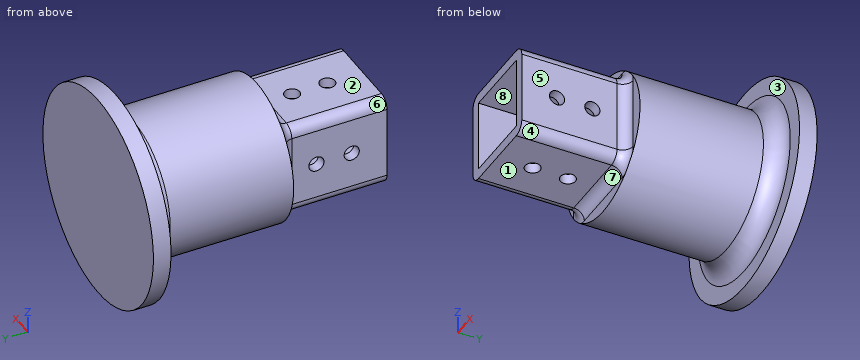
```python
from build123d import *

# Parameters (mm, degrees)
SKETCH_1_R          = 20
SKETCH_1_W          = 20.5
SKETCH_1_H          = 20.5
EXTRUDE_1_DEPTH     = 30
SKETCH_5_R          = 20
EXTRUDE_3_DEPTH     = 10
SKETCH_3_W          = 26.5
SKETCH_3_H          = 26.5
SKETCH_3_W_2        = 20.5
SKETCH_3_H_2        = 20.5
EXTRUDE_4_DEPTH     = 30
SKETCH_6_R          = 2.15
CUT_EXTRUDE_1_DEPTH = 30
SKETCH_7_R          = 2.15
CUT_EXTRUDE_2_DEPTH = 30
FILLET_1_R          = 3
FILLET_2_R          = 3
FILLET_3_R          = 3
FILLET_4_R          = 3
FILLET_5_R          = 3
SKETCH_11_R         = 30
EXTRUDE_5_DEPTH     = 5
FILLET_6_R          = 5


with BuildPart() as part:
    # 草图1 → 凸台-拉伸1 (new body)
    with BuildSketch(Plane(origin=(0, 0, 0), x_dir=(1, 0, 0), z_dir=(0, 1, 0))):
        with Locations(Location((0, 0, 0), (0, 0, 270))):
            Circle(SKETCH_1_R)
        Rectangle(SKETCH_1_W, SKETCH_1_H, mode=Mode.SUBTRACT)
    extrude(amount=EXTRUDE_1_DEPTH)

    # 草图5 → 凸台-拉伸3 (add)
    with BuildSketch(Plane(origin=(0, 30, 0), x_dir=(1, 0, 0), z_dir=(0, 1, 0))):
        with Locations(Location((0, 0, 0), (0, 0, 270))):
            Circle(SKETCH_5_R)
    extrude(amount=EXTRUDE_3_DEPTH)

    # 草图3 → 凸台-拉伸4 (add)
    with BuildSketch(Plane.XZ):
        Rectangle(SKETCH_3_W, SKETCH_3_H)
        Rectangle(SKETCH_3_W_2, SKETCH_3_H_2, mode=Mode.SUBTRACT)
    extrude(amount=EXTRUDE_4_DEPTH)

    # 草图6 → 切除-拉伸1 (cut)
    with BuildSketch(Plane.XY.offset(13.25)):
        with Locations((0, -10)):
            Circle(SKETCH_6_R)
        with Locations((0, -20)):
            Circle(SKETCH_6_R)
    extrude(amount=-CUT_EXTRUDE_1_DEPTH, mode=Mode.SUBTRACT)

    # 草图7 → 切除-拉伸2 (cut)
    with BuildSketch(Plane.ZY.offset(13.25)):
        with Locations((0, -10)):
            Circle(SKETCH_7_R)
        with Locations((0, -20)):
            Circle(SKETCH_7_R)
    extrude(amount=-CUT_EXTRUDE_2_DEPTH, mode=Mode.SUBTRACT)

    # 圆角1
    fillet_1_edges = [part.edges().sort_by_distance(p)[0] for p in [
        (-13.25, -15, 13.25),
    ]]
    fillet(fillet_1_edges, radius=FILLET_1_R)

    # 圆角2
    fillet_2_edges = [part.edges().sort_by_distance(p)[0] for p in [
        (13.25, -15, 13.25),
    ]]
    fillet(fillet_2_edges, radius=FILLET_2_R)

    # 圆角3
    fillet_3_edges = [part.edges().sort_by_distance(p)[0] for p in [
        (13.25, -15, -13.25),
    ]]
    fillet(fillet_3_edges, radius=FILLET_3_R)

    # 圆角4
    fillet_4_edges = [part.edges().sort_by_distance(p)[0] for p in [
        (-13.25, -15, -13.25),
    ]]
    fillet(fillet_4_edges, radius=FILLET_4_R)

    # 圆角5
    # the kernel refuses this fillet: 3 mm, written as the material it adds along each edge
    with BuildSketch(Plane(origin=(10.25, 0, 13.25), x_dir=(0, 0, 1), z_dir=(-1, 0, 0)), Plane(origin=(13.25, 0, -10.25), x_dir=(1, 0, 0), z_dir=(0, 0, 1)), Plane(origin=(-10.25, 0, -13.25), x_dir=(0, 0, -1), z_dir=(1, 0, 0)), Plane(origin=(-13.25, 0, 10.25), x_dir=(-1, 0, 0), z_dir=(0, 0, -1))) as fillet_5_piece_1:
        with BuildLine():
            CenterArc((FILLET_5_R, -FILLET_5_R), FILLET_5_R, 90, 90)
            Line((0, -FILLET_5_R), (0, 0))
            Line((0, 0), (FILLET_5_R, 0))
        make_face()
    extrude(amount=20.5)
    with BuildSketch(Plane(origin=(10.25, 0, 10.25), x_dir=(0, 0, 1), z_dir=(-1, 0, 0))) as fillet_5_piece_2_section:
        with BuildLine():
            CenterArc((3 + FILLET_5_R, -FILLET_5_R), FILLET_5_R, 90, 90)
            Line((3, -FILLET_5_R), (3, 0))
            Line((3, 0), (3 + FILLET_5_R, 0))
        make_face()
    fillet_5_piece_2 = revolve(axis=Axis((10.25, 0, 10.25), (0, 1, 0)), revolution_arc=90, mode=Mode.PRIVATE)
    fillet_5_piece_2 = fillet_5_piece_2 & Plane(origin=(0, -0.618331703, 0), x_dir=(0, 0, 1), z_dir=(0, -1, 0)) * Cylinder(20, 24, mode=Mode.PRIVATE)
    add(fillet_5_piece_2)
    with BuildSketch(Plane(origin=(10.25, 0, -10.25), x_dir=(1, 0, 0), z_dir=(0, 0, 1))) as fillet_5_piece_3_section:
        with BuildLine():
            CenterArc((3 + FILLET_5_R, -FILLET_5_R), FILLET_5_R, 90, 90)
            Line((3, -FILLET_5_R), (3, 0))
            Line((3, 0), (3 + FILLET_5_R, 0))
        make_face()
    fillet_5_piece_3 = revolve(axis=Axis((10.25, 0, -10.25), (0, 1, 0)), revolution_arc=90, mode=Mode.PRIVATE)
    fillet_5_piece_3 = fillet_5_piece_3 & Plane(origin=(0, -0.618331703, 0), x_dir=(0, 0, 1), z_dir=(0, -1, 0)) * Cylinder(20, 24, mode=Mode.PRIVATE)
    add(fillet_5_piece_3)
    with BuildSketch(Plane(origin=(-10.25, 0, -10.25), x_dir=(0, 0, -1), z_dir=(1, 0, 0))) as fillet_5_piece_4_section:
        with BuildLine():
            CenterArc((3 + FILLET_5_R, -FILLET_5_R), FILLET_5_R, 90, 90)
            Line((3, -FILLET_5_R), (3, 0))
            Line((3, 0), (3 + FILLET_5_R, 0))
        make_face()
    fillet_5_piece_4 = revolve(axis=Axis((-10.25, 0, -10.25), (0, 1, 0)), revolution_arc=90, mode=Mode.PRIVATE)
    fillet_5_piece_4 = fillet_5_piece_4 & Plane(origin=(0, -0.618331703, 0), x_dir=(0, 0, 1), z_dir=(0, -1, 0)) * Cylinder(20, 24, mode=Mode.PRIVATE)
    add(fillet_5_piece_4)
    with BuildSketch(Plane(origin=(-10.25, 0, 10.25), x_dir=(-1, 0, 0), z_dir=(0, 0, -1))) as fillet_5_piece_5_section:
        with BuildLine():
            CenterArc((3 + FILLET_5_R, -FILLET_5_R), FILLET_5_R, 90, 90)
            Line((3, -FILLET_5_R), (3, 0))
            Line((3, 0), (3 + FILLET_5_R, 0))
        make_face()
    fillet_5_piece_5 = revolve(axis=Axis((-10.25, 0, 10.25), (0, 1, 0)), revolution_arc=90, mode=Mode.PRIVATE)
    fillet_5_piece_5 = fillet_5_piece_5 & Plane(origin=(0, -0.618331703, 0), x_dir=(0, 0, 1), z_dir=(0, -1, 0)) * Cylinder(20, 24, mode=Mode.PRIVATE)
    add(fillet_5_piece_5)

    # 草图11 → 凸台-拉伸5 (add)
    with BuildSketch(Plane(origin=(0, 40, 0), x_dir=(1, 0, 0), z_dir=(0, 1, 0))):
        with Locations(Location((0, 0, 0), (0, 0, 270))):
            Circle(SKETCH_11_R)
    extrude(amount=EXTRUDE_5_DEPTH)

    # 圆角6
    fillet_6_edges = [part.edges().sort_by_distance(p)[0] for p in [
        (0, 40, -20),
    ]]
    fillet(fillet_6_edges, radius=FILLET_6_R)


solid = part.part
```
Here's how the part is built. I have some questions about the finished solid (model axes, mm). Face numbers are marked on the shaded views. A direction names the side the tool comes from. Coordinates: 2 decimals unless noted, no trailing zeros. Loops run counter-clockwise (first coordinate to the right, second up) from the corner with the lowest first, then second, coordinate; pieces in that order, holes last. Notation, with made-up numbers: (-39, 65) - (5, 65) arc R21 cw to (5, 94) - close; hole circle Ø3 at (-34, -20). An arc over 180 degrees is marked (long way). Return JSON: item names as keys, results as strings. Group by question number.
Item 1: If we section it at B-B on y = 19: Write out the boundary of the cut face in (x, z), and give its area (3 significant figures).
Item 2: I need wall thicknesses on line 1 (Y direction, x = -12, z = 0); line 2 (Z direction, x = -5.5, y = -10.5); line 3 (Y direction, x = 21.5, z = -20). Which ranges of each line are inside material? Lowest first, please. Write a range as from..to.
Item 3: Will these pins go through, and if not, where does the flat tip stop? P1, Ø1.5, axis at x = -1.5, z = -20, coming from the -Y side; P2, Ø2.5, axis at x = 0, y = -20, coming from the -Z side; P3, Ø22.5, axis at x = 1, y = -10, coming from the +Z side; P4, Ø5, axis at x = -22, z = -23.5, coming from the -Y side.
Item 4: If we section it at C-C on x = 0: State how many separate pieces and enclosed holes the cut face has, and give its area (3 significant figures).
Item 5: On a 3-axis mill with a long thin cutter (end or side, diameter ignored), from which of +Z, -Z, +X, -X, +Y, -Y can I reach the whole of each face in a straight line? I mean the marked faces 1, 2, 3, 4 and 5. Say none if no direction works.
Item 6: If we section it at A-A on y = -10: Write out the boundary of the cut face in (x, z), and give its area (3 significant figures).
Item 7: We'd pull the mould along X, two halves only. Please class the marked faces 6, 7 and 8: +X half, -X half, draft (parallel to the pull), parting line (faces both ways), or undercut.
Calculated:
{
 "1": {"outline": "circle Ø40 at (0, 0); hole (-10.25, -10.25) - (10.25, -10.25) - (10.25, 10.25) - (-10.25, 10.25) - close", "area": "836 mm^2"},
 "2": {"line 1": "y = -30..-22.15, -17.85..-12.15, -7.85..45", "line 2": "z = -13.25..-10.25, 10.25..13.25", "line 3": "y = 40..45"},
 "3": {"P1": "stops at y = 0", "P2": "passes through", "P3": "stops at z = 20", "P4": "stops at y = 40"},
 "4": {"separate pieces": "5", "enclosed holes": "0", "area": "1,430 mm^2"},
 "5": {"face 1": "-Z, +X, -X, -Y", "face 2": "+Z, +X, -X, -Y", "face 3": "-Y", "face 4": "-Z, +X, -Y", "face 5": "+Z, -Z, +X, -Y"},
 "6": {"outline": "(-13.25, -10.25) arc R3 ccw to (-10.25, -13.25) - (-2.15, -13.25) - (-2.15, -10.25) - (-10.25, -10.25) - (-10.25, -2.15) - (-13.25, -2.15) - close; (-13.25, 2.15) - (-10.25, 2.15) - (-10.25, 10.25) - (-2.15, 10.25) - (-2.15, 13.25) - (-10.25, 13.25) arc R3 ccw to (-13.25, 10.25) - close; (2.15, -13.25) - (10.25, -13.25) arc R3 ccw to (13.25, -10.25) - (13.25, -2.15) - (10.25, -2.15) - (10.25, -10.25) - (2.15, -10.25) - close; (2.15, 10.25) - (10.25, 10.25) - (10.25, 2.15) - (13.25, 2.15) - (13.25, 10.25) arc R3 ccw to (10.25, 13.25) - (2.15, 13.25) - close", "area": "223 mm^2"},
 "7": {"face 6": "-X half", "face 7": "draft", "face 8": "undercut"}
}
